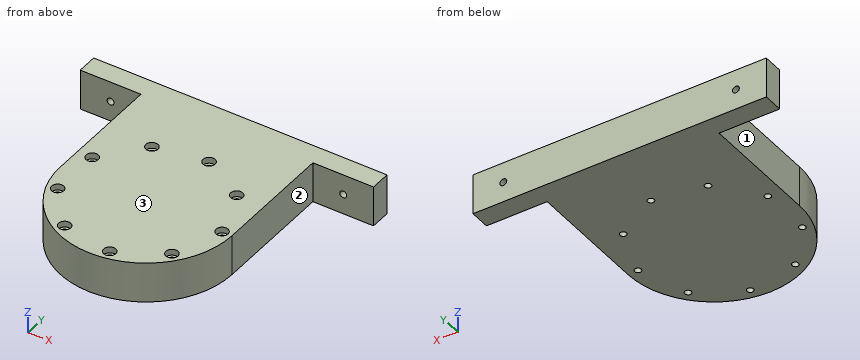
```python
from build123d import *

# Parameters (mm, degrees)
SKETCH1_R           = 1.6
BOSS_EXTRUDE2_DEPTH = 20
SKETCH2_R           = 3
CUT_EXTRUDE1_DEPTH  = 3
SKETCH3_R           = 1.7
CUT_EXTRUDE2_DEPTH  = 128.131821351


with BuildPart() as part:
    # Sketch1 → Boss-Extrude2 (new body)
    with BuildSketch(Plane.XY):
        with BuildLine():
            Line((-42.5, 0), (-42.5, 60))
            Line((-42.5, 60), (-72.5, 60))
            Line((-72.5, 60), (-72.5, 70))
            Line((-72.5, 70), (72.5, 70))
            Line((72.5, 70), (72.5, 60))
            Line((72.5, 60), (42.5, 60))
            Line((42.5, 60), (42.5, 0))
            ThreePointArc((42.5, 0), (0, -42.5), (-42.5, 0))
        make_face()
        with Locations((37.5, 0)):
            Circle(SKETCH1_R, mode=Mode.SUBTRACT)
        with Locations((28.726666617, -24.104535363)):
            Circle(SKETCH1_R, mode=Mode.SUBTRACT)
        with Locations((6.511806663, -36.930290738)):
            Circle(SKETCH1_R, mode=Mode.SUBTRACT)
        with Locations((-18.75, -32.475952642)):
            Circle(SKETCH1_R, mode=Mode.SUBTRACT)
        with Locations((-35.238473279, -12.825755375)):
            Circle(SKETCH1_R, mode=Mode.SUBTRACT)
        with Locations((-35.238473279, 12.825755375)):
            Circle(SKETCH1_R, mode=Mode.SUBTRACT)
        with Locations((-18.75, 32.475952642)):
            Circle(SKETCH1_R, mode=Mode.SUBTRACT)
        with Locations((6.511806663, 36.930290738)):
            Circle(SKETCH1_R, mode=Mode.SUBTRACT)
        with Locations((28.726666617, 24.104535363)):
            Circle(SKETCH1_R, mode=Mode.SUBTRACT)
    extrude(amount=BOSS_EXTRUDE2_DEPTH)

    # Sketch2 → Cut-Extrude1 (cut)
    with BuildSketch(Plane.XY.offset(20)):
        with Locations((6.511806663, 36.930290738)):
            Circle(SKETCH2_R)
        with Locations((28.726666617, 24.104535363)):
            Circle(SKETCH2_R)
        with Locations((37.5, 0)):
            Circle(SKETCH2_R)
        with Locations((28.726666617, -24.104535363)):
            Circle(SKETCH2_R)
        with Locations((6.511806663, -36.930290738)):
            Circle(SKETCH2_R)
        with Locations((-18.75, -32.475952642)):
            Circle(SKETCH2_R)
        with Locations((-35.238473279, -12.825755375)):
            Circle(SKETCH2_R)
        with Locations((-35.238473279, 12.825755375)):
            Circle(SKETCH2_R)
        with Locations((-18.75, 32.475952642)):
            Circle(SKETCH2_R)
    extrude(amount=-CUT_EXTRUDE1_DEPTH, mode=Mode.SUBTRACT)

    # Sketch3 → Cut-Extrude2 (cut, through all)
    with BuildSketch(Plane.XZ.offset(-60)):
        with Locations(Location((57.5, 10, 0), (0, 0, 270))):
            Circle(SKETCH3_R)
        with Locations(Location((-57.5, 10, 0), (0, 0, 270))):
            Circle(SKETCH3_R)
    extrude(amount=-CUT_EXTRUDE2_DEPTH, mode=Mode.SUBTRACT)


solid = part.part
```
Design review of the part built by this model. Coordinates are the model's own, in mm. Face numbers are marked on the shaded views. A direction names the side the tool comes from. Coordinates: 2 decimals unless noted, no trailing zeros. Write each loop counter-clockwise with the first axis right and the second up, starting at its lowest first coordinate (ties: lowest second). Pieces come first, ordered by that corner, then holes.
1) Machinability: for the marked faces 1, 2 and 3, which of the approach directions +Z, -Z, +X, -X, +Y, -Y give a long, thin tool a straight path to every point of the face, cutting with its end or side? Answer none if there is none.
2) Add section A-A (x = -57.5). Write out the cut boundary in (y, z), plus the area to 3 significant figures.
3) Add section B-B (z = 10). State how many separate pieces and enclosed holes the cut face has, plus the area to 3 significant figures.
4) Add section C-C (x = -18.75). Write out the cut boundary in (y, z).
5) Insertion check: pin 1 (3.5 mm diameter, centred on x = -18.75, y = 32.48, fed in from +Z); pin 2 (1.8 mm diameter, centred on x = 28.5, y = -24, fed in from +Z); pin 3 (2 mm diameter, centred on y = -8, z = 3, fed in from -X); pin 4 (6 mm diameter, centred on x = 34.5, z = 4.5, fed in from -Y). Each pin has a flat end and moves straight along its axis. Give the tip position at first contact, or say it passes through.
6) To check wall thickness, follow L1, parallel to X at y = 66.75, z = 10; L2, parallel to Y at x = -18.75, z = 8.5; L3, parallel to Y at x = -1, z = 19.25. State the ranges of each line that lie inside material, in increasing order.
Check result:
1. face 1: +Z, -Z, -X, -Y
1. face 2: +Z, -Z, +X, -Y
1. face 3: +Z, +X, -X, +Y, -Y
2. outline: (60, 0) - (70, 0) - (70, 8.3) - (60, 8.3) - close; (60, 11.7) - (70, 11.7) - (70, 20) - (60, 20) - close
2. area: 166 mm2
3. separate pieces: 3
3. enclosed holes: 9
3. area: 9,250 mm2
4. outline: (-38.14, 0) - (-34.08, 0) - (-34.08, 17) - (-35.48, 17) - (-35.48, 20) - (-38.14, 20) - close; (-30.88, 0) - (30.88, 0) - (30.88, 17) - (29.48, 17) - (29.48, 20) - (-29.48, 20) - (-29.48, 17) - (-30.88, 17) - close; (34.08, 0) - (70, 0) - (70, 20) - (35.48, 20) - (35.48, 17) - (34.08, 17) - close
5. pin 1: stops at z = 17
5. pin 2: passes through
5. pin 3: stops at x = -41.92
5. pin 4: stops at y = -28.53
6. L1: x = -72.5 to -59.2, -55.8 to 55.8, 59.2 to 72.5
6. L2: y = -38.14 to -34.08, -30.88 to 30.88, 34.08 to 70
6. L3: y = -42.49 to 70
